The drawing under review shows one solid part. Ordinate dimensions are in mm from its lowest x, y, z. A direction names the side the tool comes from. Coordinates: 2 decimals unless noted, no trailing zeros. Write each loop counter-clockwise with the first axis right and the second up, starting at its lowest first coordinate (ties: lowest second). Pieces come first, ordered by that corner, then holes. Notation, with made-up numbers: M 57.5,-8.75 L 102.5,-8.75 A13 ccw 102.5,-1.75 Z; hole C 79.5,72.25 d1. An arc over 180 degrees is marked long. Write item = value, one per line.
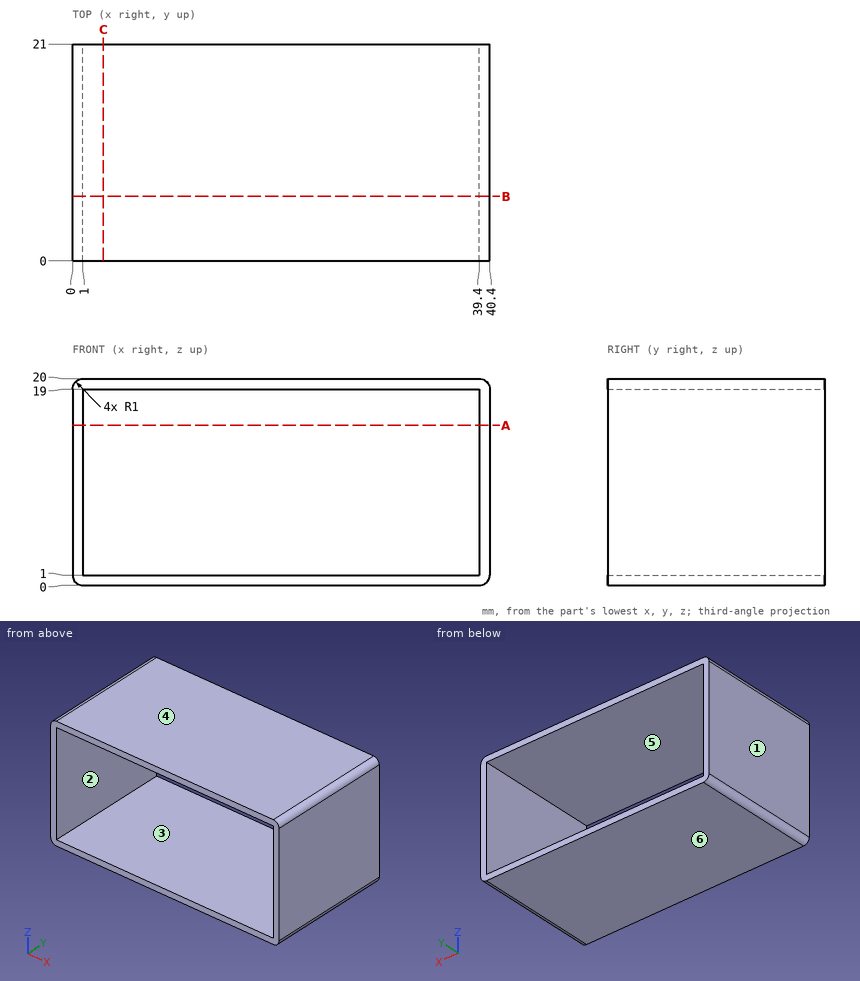
Q1. Machinability: for the marked faces 5 and 6, which of the approach directions +Z, -Z, +X, -X, +Y, -Y give a long, thin tool a straight path to every point of the face, cutting with its end or side? Answer none if there is none.
Check result:
face_5 = +Y, -Y
face_6 = -Z, +X, -X, +Y, -Y
Q2. Consider section A-A, the plane z = 15.5. State the section outline as (x, y) points, and give its area (3 significant figures).
Check result:
outline = M 0,0 L 1,0 L 1,21 L 0,21 Z; M 39.4,0 L 40.4,0 L 40.4,21 L 39.4,21 Z
area = 42.0 mm²
Q3. The part is to be moulded in two halves that separate along X. For the marked faces 1, 2, 3 and 4, say which applies: +X half, -X half, draft (parallel to the pull), parting line (faces both ways), or undercut.
Check result:
face_1 = -X half
face_2 = undercut
face_3 = undercut
face_4 = draft
Q4. Consider section B-B, the plane y = 6.25. State the section outline as (x, z) points, and give its area (3 significant figures).
Check result:
outline = M 0,1 A1 ccw 1,0 L 39.4,0 A1 ccw 40.4,1 L 40.4,19 A1 ccw 39.4,20 L 1,20 A1 ccw 0,19 Z; hole M 1,1 L 39.4,1 L 39.4,19 L 1,19 Z
area = 116 mm²
Q5. Consider section C-C, the plane x = 3. State the section outline as (y, z) points, and give its area (3 significant figures).
Check result:
outline = M 0,0 L 21,0 L 21,1 L 0,1 Z; M 0,19 L 21,19 L 21,20 L 0,20 Z
area = 42.0 mm²
Q6. Wall thickness on line 1 (Z direction, x = 31, y = 5.5); line 2 (X direction, y = 18, z = 14.5): over which ranges is each line inside the solid? List them lowest first.
Check result:
line_1 = 0 to 1, 19 to 20
line_2 = 0 to 1, 39.4 to 40.4
